Geometry check sheet. Reference: the model listing, model coordinates, mm. A direction names the side the tool comes from. Coordinates: 2 decimals unless noted, no trailing zeros. Loops run counter-clockwise (first coordinate to the right, second up) from the corner with the lowest first, then second, coordinate; pieces in that order, holes last. Notation, with made-up numbers: (-10.5, 5.5) - (0.5, 5.5) arc R22 cw to (0.5, 31.5) - close; hole circle Ø5 at (-34.75, 66). An arc over 180 degrees is marked (long way). Write each question's results on one line, items separated by ' | '. Start each with the question number.
(1) Access from +Z, -Z, +X, -X, +Y, -Y to the whole of each face (thin tool, end or side, straight path). Record for faces 1 (the face through (20, -6.17, 1)), 2 (the face through (-17, -6.17, 2)), 3 (the face through (-8.916, -19, 2)).
(2) Sectioned sample at A-A (z = 2.5). Enter the section's corners in (x, y).
(3) Go/stop test with flat-tipped pins: pin 1 Ø1.5 at (y, z) = (-19.5, 3.5) entering from +X; pin 2 Ø1 at (x, z) = (-16.5, 4) entering from -Y; pin 3 Ø2.5 at (x, z) = (21.08, 2.5) entering from -Y; pin 4 Ø1.5 at (x, z) = (-19, 1.5) entering from +Y. Record where each tip stops, or that it passes through.
(4) Material ranges on probe 1 along X at (y, z) = (13, 0.65); probe 2 along X at (y, z) = (14.5, 3.55); probe 3 along Y at (x, z) = (1, 3.5), recorded low to high.
(5) Sectioned sample at C-C (y = 5.5). Enter the section's corners in (x, z), plus the area to 3 significant figures.
(6) Mould release check, pull along X, two halves, no side actions. Record for faces 4 (the face through (22.5, -11.1, 2)), 5 (the face through (-24.916, -11, 2)), 6 (the face through (1, 1, 0)): pulls with the +X half, pulls with the -X half, needs draft (parallel to the pull), parting line crosses it, or undercut.
(7) Sectioned sample at B-B (x = 17). Enter the section's corners in (y, z).
from build123d import *

# Parameters (mm, degrees)
SKETCH1_R           = 3
SKETCH1_R_2         = 1.5
BOSS_EXTRUDE1_DEPTH = 5
SKETCH2_R           = 1.5
CUT_EXTRUDE1_DEPTH  = 10
SKETCH2_3_R         = 1.5
CUT_EXTRUDE2_DEPTH  = 10


with BuildPart() as part:
    # Sketch1 → Boss-Extrude1 (new body)
    with BuildSketch(Plane.XY):
        Polygon((12.083913986, -6.170151075), (12.083913986, 21.829848925), (-9.916086014, 21.829848925), (-9.916086014, -6.170151075), (-24.916086014, -6.170151075), (-24.916086014, -16.170151075), (-8.916086014, -16.170151075), (-8.916086014, -21.170151075), (11.083913986, -21.170151075), (11.083913986, -16.170151075), (27.083913986, -16.170151075), (27.083913986, -6.170151075), align=None)
        with Locations((1.083913986, -6.170151075)):
            Circle(SKETCH1_R, mode=Mode.SUBTRACT)
        with Locations((-7.416086014, 13.829848925)):
            Circle(SKETCH1_R_2, mode=Mode.SUBTRACT)
        with Locations(Location((9.583913986, 13.829848925, 0), (0, 0, 180))):
            Circle(SKETCH1_R_2, mode=Mode.SUBTRACT)
    extrude(amount=BOSS_EXTRUDE1_DEPTH)

    # Sketch2 → Cut-Extrude1 (cut)
    with BuildSketch(Plane(origin=(0, -6.170151075, 0), x_dir=(1, 0, 0), z_dir=(0, 1, 0))):
        with Locations(Location((-18.916086014, -2.5, 0), (0, 0, 180))):
            Circle(SKETCH2_R)
    extrude(amount=-CUT_EXTRUDE1_DEPTH, mode=Mode.SUBTRACT)

    # Sketch2_3 → Cut-Extrude2 (cut)
    with BuildSketch(Plane(origin=(0, -6.170151075, 0), x_dir=(1, 0, 0), z_dir=(0, 1, 0))):
        with Locations(Location((-18.916086014, -2.5, 0), (0, 0, 180))):
            Circle(SKETCH2_3_R)
        with Locations((21.083913986, -2.5)):
            Circle(SKETCH2_3_R)
    extrude(amount=-CUT_EXTRUDE2_DEPTH, mode=Mode.SUBTRACT)


solid = part.part
Outcome:
1) face 1: +Z, -Z, +X, +Y | face 2: +Z, -Z, -X, +Y | face 3: +Z, -Z, -X, -Y
2) outline: (-24.92, -16.17) - (-20.42, -16.17) - (-20.42, -6.17) - (-24.92, -6.17) - close; (-17.42, -16.17) - (-8.92, -16.17) - (-8.92, -21.17) - (11.08, -21.17) - (11.08, -16.17) - (19.58, -16.17) - (19.58, -6.17) - (12.08, -6.17) - (12.08, 21.83) - (-9.92, 21.83) - (-9.92, -6.17) - (-17.42, -6.17) - close; (22.58, -16.17) - (27.08, -16.17) - (27.08, -6.17) - (22.58, -6.17) - close; hole circle Ø3 at (-7.42, 13.83); hole circle Ø6 at (1.08, -6.17); hole circle Ø3 at (9.58, 13.83)
3) pin 1: stops at x = 11.08 | pin 2: stops at y = -16.17 | pin 3: passes through | pin 4: stops at y = -6.17
4) probe 1: x = -9.92 to -8.67, -6.17 to 8.33, 10.83 to 12.08 | probe 2: x = -9.92 to -8.76, -6.07 to 8.24, 10.93 to 12.08 | probe 3: y = -21.17 to -9.17, -3.17 to 21.83
5) outline: (-9.92, 0) - (12.08, 0) - (12.08, 5) - (-9.92, 5) - close | area: 110 mm2
6) face 4: undercut | face 5: pulls with the -X half | face 6: needs draft
7) outline: (-16.17, 0) - (-6.17, 0) - (-6.17, 5) - (-16.17, 5) - close
